from build123d import *

# Parameters (mm, degrees)
BOSS_EXTRUDE1_DEPTH = 3.175
FILLET1_R           = 10
SKETCH2_R           = 1.7
SKETCH2_R_2         = 1.45
CUT_EXTRUDE1_DEPTH  = 3.175
SKETCH6_W           = 49.8
SKETCH6_H           = 2.6
CUT_EXTRUDE2_DEPTH  = 3.175


with BuildPart() as part:
    # Sketch1 → Boss-Extrude1 (new body)
    with BuildSketch(Plane(origin=(0, 0, 0), x_dir=(1, 0, 0), z_dir=(0, 1, 0))):
        Polygon((0, 240), (0, 60), (80, 0), (340, 0), (420, 60), (420, 240), align=None)
    extrude(amount=BOSS_EXTRUDE1_DEPTH)

    # Fillet1
    fillet1_edges = [part.edges().sort_by_distance(p)[0] for p in [
        (420, 1.5875, -240),
        (420, 1.5875, -60),
        (340, 1.5875, 0),
        (80, 1.5875, 0),
        (0, 1.5875, -60),
        (0, 1.5875, -240),
    ]]
    fillet(fillet1_edges, radius=FILLET1_R)

    # Sketch2 → Cut-Extrude1 (cut)
    with BuildSketch(Plane(origin=(0, 3.175, 0), x_dir=(1, 0, 0), z_dir=(0, 1, 0))):
        with Locations(Location((11, 229, 0), (0, 0, 270))):
            Circle(SKETCH2_R)
        with Locations(Location((11, 65.5, 0), (0, 0, 270))):
            Circle(SKETCH2_R)
        with Locations(Location((83.666666667, 11, 0), (0, 0, 270))):
            Circle(SKETCH2_R)
        with Locations(Location((409, 65.5, 0), (0, 0, 270))):
            Circle(SKETCH2_R)
        with Locations(Location((336.333333333, 11, 0), (0, 0, 270))):
            Circle(SKETCH2_R)
        with Locations(Location((210, 115, 0), (0, 0, 270))):
            Circle(SKETCH2_R_2)
        with Locations(Location((132, 115, 0), (0, 0, 270))):
            Circle(SKETCH2_R_2)
        with Locations(Location((288, 115, 0), (0, 0, 270))):
            Circle(SKETCH2_R_2)
        with Locations(Location((40, 222.825, 0), (0, 0, 270))):
            Circle(SKETCH2_R)
        with Locations(Location((380, 222.825, 0), (0, 0, 270))):
            Circle(SKETCH2_R)
        with Locations(Location((409, 229, 0), (0, 0, 270))):
            Circle(SKETCH2_R)
    extrude(amount=-CUT_EXTRUDE1_DEPTH, mode=Mode.SUBTRACT)

    # Sketch6 → Cut-Extrude2 (cut)
    with BuildSketch(Plane(origin=(0, 3.175, 0), x_dir=(1, 0, 0), z_dir=(0, 1, 0))):
        with Locations((160, 6.5875)):
            Rectangle(SKETCH6_W, SKETCH6_H)
        with Locations((125, 230.4125)):
            Rectangle(SKETCH6_W, SKETCH6_H)
        with Locations((295, 230.4125)):
            Rectangle(SKETCH6_W, SKETCH6_H)
        with Locations((260, 6.5875)):
            Rectangle(SKETCH6_W, SKETCH6_H)
    extrude(amount=-CUT_EXTRUDE2_DEPTH, mode=Mode.SUBTRACT)


solid = part.part
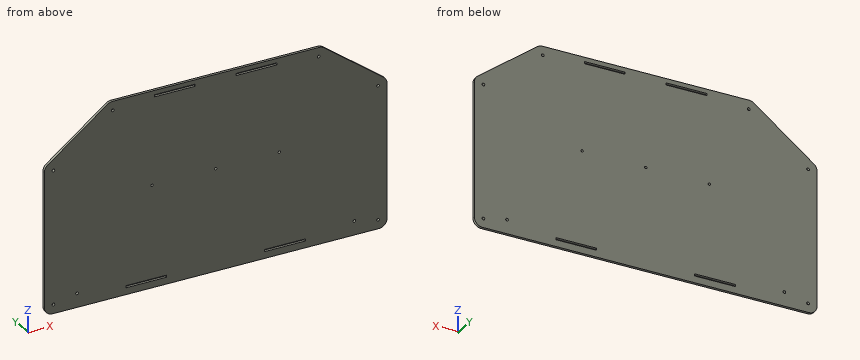
Here's how the part is built. I have some questions about the finished solid (model axes, mm). Give positions to 0.01 mm unless a question says otherwise; leave off trailing zeros. Write each loop counter-clockwise with the first axis right and the second up, starting at its lowest first coordinate (ties: lowest second). Pieces come first, ordered by that corner, then holes. Notation, with made-up numbers: (45.5, -33.5) -> (69.5, -33.5) arc R13 ccw to (69.5, -29.5) -> close; hole circle Ø3 at (-39.5, 18). An arc over 180 degrees is marked (long way). Use one line per item in the form item = value. Start each with the question number.
1. Imagine slicing it at B-B on x = 55. List the corners of the cut face in (y, z) for me (3 decimals), plus the area to 3 significant figures.
2. Imagine slicing it at A-A on z = -30. List the corners of the cut face in (x, y) for me (3 decimals).
3. Will these pins go through, and if not, where does the flat tip stop? pin 1 Ø2.5 at (x, z) = (11, -65.5) entering from +Y; pin 2 Ø1.3 at (y, z) = (2, -6) entering from +X.
4. Imagine slicing it at C-C on y = 2.3. State how many separate pieces and enclosed holes the cut face has, plus the area to 3 significant figures.
5. If I drill on L1, parallel to Z at x = 288, y = 1.05; L2, parallel to Z at x = 276, y = 0.65; L3, parallel to Z at x = 290, y = 0.4, over which ranges is the centre line in solid material (lowest first)?
Entries:
q1.outline = (0, -240) -> (3.175, -240) -> (3.175, -18.75) -> (0, -18.75) -> close
q1.area = 702 mm²
q2.outline = (40, 0) -> (380, 0) -> (380, 3.175) -> (40, 3.175) -> close
q3.pin_1 = through
q3.pin_2 = 348.87
q4.separate_pieces = 1
q4.enclosed_holes = 15
q4.area = 95,300 mm²
q5.L1 = -240 to -231.71, -229.11 to -116.45, -113.55 to 0
q5.L2 = -240 to -231.71, -229.11 to -7.89, -5.29 to 0
q5.L3 = -240 to -231.71, -229.11 to 0
